Autodesk Fusion 360 part; units mm, degrees
sketch "草图1" plane through (0, 0, 0) normal (0, 1, 0) x (1, 0, 0)
  line L0 (2.4024, -17.839) -> (16.6502, 6.839)
  line L1 (-16.6502, 6.839) -> (-2.4024, -17.839)
  arc A0 (-14.2478, 11) -> (-16.6502, 6.839) centre (0, 0) ccw
  line L2 (14.2478, 11) -> (-14.2478, 11)
  arc A1 (16.6502, 6.839) -> (14.2478, 11) centre (0, 0) ccw
  arc A2 (-2.4024, -17.839) -> (2.4024, -17.839) centre (0, 0) ccw
  line L3 (12.1244, 7) -> (-12.1244, 7)
  line L4 (-12.1244, 7) -> (0, -14)
  line L5 (0, -14) -> (12.1244, 7)
  line L6 (0, -14) -> (1.1374, -0.6567)
  line L7 (12.1244, 7) -> (1.1374, -0.6567)
  line L8 (1.3775, -9.6141) -> (2.0939, -1.2089)
  line L9 (9.0148, 3.6141) -> (2.0939, -1.2089)
  line L10 (2.047, -1.7592) -> (4.9462, -3.433)
  line L11 (2.547, -0.8932) -> (5.4462, -2.567)
  line L12 (1.3775, -9.6141) -> (4.9462, -3.433)
  line L13 (5.4462, -2.567) -> (9.0148, 3.6141)
  line L14 (12.1244, 7) -> (0, 1.3134)
  line L15 (7.6373, 6) -> (0, 2.4179)
  line L16 (0.5, 2.6524) -> (0.5, 6)
  line L17 (-0.5, 2.6524) -> (-0.5, 6)
  line L18 (-7.6373, 6) -> (0, 2.4179)
  line L19 (-12.1244, 7) -> (0, 1.3134)
  line L20 (-0.5, 6) -> (-7.6373, 6)
  line L21 (7.6373, 6) -> (0.5, 6)
  line L22 (-12.1244, 7) -> (-1.1374, -0.6567)
  line L23 (-9.0148, 3.6141) -> (-2.0939, -1.2089)
  line L24 (-2.547, -0.8932) -> (-5.4462, -2.567)
  line L25 (-2.047, -1.7592) -> (-4.9462, -3.433)
  line L26 (-1.3775, -9.6141) -> (-2.0939, -1.2089)
  line L27 (0, -14) -> (-1.1374, -0.6567)
  line L28 (-4.9462, -3.433) -> (-1.3775, -9.6141)
  line L29 (-9.0148, 3.6141) -> (-5.4462, -2.567)
  circle A3 centre (0, -14) radius 2.5
  circle A4 centre (12.1244, 7) radius 2.5
  circle A5 centre (-12.1244, 7) radius 2.5
  dimension "d1" = -4
  dimension "d6" = 360
  dimension "d7" = 5
  dimension "d9" = 360
extrude "拉伸1" add sketch "草图1" along normal blind 1 contours L3 L19 A5 | L3 L14 L19 A4 A5 | L4 L22 A5 | L19 L22 A5 | L3 L14 A4 | L4 L22 L27 A3 A5 | L5 L7 A4 | L7 L14 A4 | L4 L27 A3 | L5 L6 L7 A3 A4 | L5 L6 A3 | L6 L27 A3
Can you work these out from the model? Positions are in its coordinate system, mm. A direction names the side the tool comes from. Coordinates: 2 decimals unless noted, no trailing zeros. Loops run counter-clockwise (first coordinate to the right, second up) from the corner with the lowest first, then second, coordinate; pieces in that order, holes last. Notation, with made-up numbers: (-6, 60.5) -> (42, 60.5) arc R32 cw to (42, 92.5) -> close; hole circle Ø7 at (-31, 7.25). An arc over 180 degrees is marked (long way). Put each result on its own line as item: value. Start each with the question number.
Q1. I want a section at C-C (z = 10). Write out the boundary of the cut face in (x, y).
Q2. Thinking about a two-plate mould opening in X: for faces 3 (the face through (4.12, 0.49, -4.35)), 4 (the face through (0.2, 0.5, -7)), 5 (the face through (5.977, 0.493, 3.647)), which applies, pulls with the +X half, pulls with the -X half, needs draft (parallel to the pull), parting line crosses it, or undercut?
Q3. I want a section at D-D (y = 0.6). Count the separate pieces of the cut face and the enclosed holes in it, plus the area to 3 significant figures.
Q4. I want a section at A-A (z = -0.25). Write out the boundary of the cut face in (x, y), plus the area to 3 significant figures.
Q5. If I drill on line 1 (Z direction, x = 4.5, y = 0.55); line 2 (Z direction, x = 8, y = 0.65); line 3 (Z direction, x = 6.25, y = 0.2), over which ranges is the centre line in solid material (lowest first)? Write a range as [from, to].
Q6. I'm going to push flat-ended pins straight in: P1, Ø12, axis at x = 0, z = 3.5, coming from the +Y side; P2, Ø1, axis at x = 6, z = 8, coming from the +Y side; P3, Ø0.5, axis at y = 0.5, z = -5, coming from the +X side. Where does each tip first touch, or does it pass through?
Q7. I want a section at B-B (x = -9.5). Write out the boundary of the cut face in (y, z), plus the area to 3 significant figures.
Q8. For faces 1 (the face through (-6.15, 0.49, 3.35)), 2 (the face through (5.826, 0.493, -1.392)), which set-ups out of +Z, -Z, +X, -X, +Y, -Y let a thin tool reach every point of the face, with its end or its side?
Taken from the geometry:
1. outline: (-2.31, 0) -> (-0.34, 0) -> (-0.34, 1) -> (-2.31, 1) -> close; (0.34, 0) -> (2.31, 0) -> (2.31, 1) -> (0.34, 1) -> close
2. face 3: undercut
2. face 4: needs draft
2. face 5: pulls with the +X half
3. separate pieces: 1
3. enclosed holes: 7
3. area: 137 mm2
4. outline: (-8.23, 0) -> (-7.07, 0) -> (-7.07, 1) -> (-8.23, 1) -> close; (-4.19, 0) -> (-2.44, 0) -> (-2.44, 1) -> (-4.19, 1) -> close; (2.44, 0) -> (4.19, 0) -> (4.19, 1) -> (2.44, 1) -> close; (7.07, 0) -> (8.23, 0) -> (8.23, 1) -> (7.07, 1) -> close
4. area: 5.81 mm2
5. line 1: z = [-7, -6], [-4.53, -3.42], [-1.69, -0.47], [2.02, 3.18], [4.21, 6.21]
5. line 2: z = [-7, -5.07], [-4.13, -2.91], [-1.86, 0.14]
5. line 3: z = [-7, -6], [-5.35, -4.24], [-2.91, -1.69], [1.17, 3.17]
6. P1: stops at y = 1
6. P2: passes through
6. P3: stops at x = 11.11
7. outline: (0, -7) -> (1, -7) -> (1, -5.77) -> (0, -5.77) -> close; (0, -5.17) -> (1, -5.17) -> (1, -2.45) -> (0, -2.45) -> close
7. area: 3.95 mm2
8. face 1: +Z, -X, +Y, -Y
8. face 2: +Y, -Y
